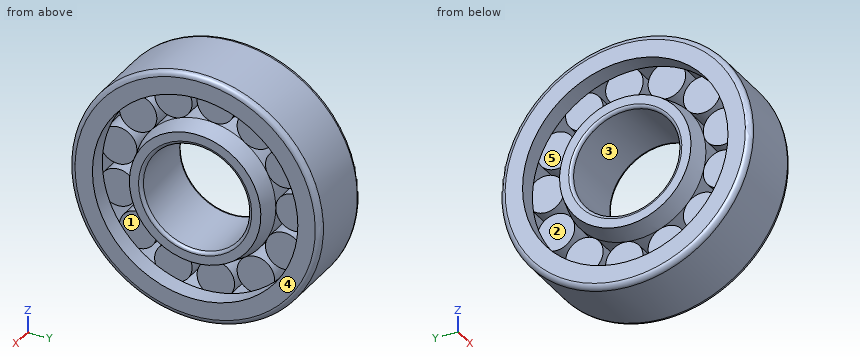
from build123d import *

# Parameters (mm, degrees)
SKETCH2_W               = 7
SKETCH2_H               = 3.51
CIRCULAR_PATTERN1_COUNT = 13
FILLET1_R               = 1
FILLET2_R               = 0.6


with BuildPart() as part:
    # Sketch1 → Revolve1 (revolve)
    with BuildSketch(Plane.XY, mode=Mode.PRIVATE) as revolve1_sk:
        Polygon((-7, 10), (7, 10), (7, 12.312177826), (3.5, 13.25), (-3.5, 13.25), (-7, 12.312177826), align=None)
    revolve(revolve1_sk.sketch.rotate(Axis((-10.137871204, 0, 0), (1, 0, 0)), 90), axis=Axis((-10.137871204, 0, 0), (1, 0, 0)))

    # Sketch2 → Revolve2 (revolve)
    with BuildSketch(Plane.XY):
        with Locations((0, 14.995)):
            Rectangle(SKETCH2_W, SKETCH2_H)
    revolve2 = revolve(axis=Axis((-7.422783257, 16.75, 0), (1, 0, 0)))

    # Sketch3 → Revolve3 (revolve)
    with BuildSketch(Plane.XY, mode=Mode.PRIVATE) as revolve3_sk:
        Polygon((-7, 23.5), (7, 23.5), (7, 19.2375), (3.49, 19.2375), (3.49, 20.25), (-3.49, 20.25), (-3.49, 19.2375), (-7, 19.2375), align=None)
    revolve(revolve3_sk.sketch.rotate(Axis((-9.082213196, 0, 0), (1, 0, 0)), 90), axis=Axis((-9.082213196, 0, 0), (1, 0, 0)))

    # Circular-Pattern1: Revolve2 ×13 about axis
    circular_pattern1_axis = Axis((0, 0, 0), (1, 0, 0))
    for i in range(1, CIRCULAR_PATTERN1_COUNT):
        add(revolve2.rotate(circular_pattern1_axis, i * 360 / CIRCULAR_PATTERN1_COUNT))

    # Fillet1
    fillet1_edges = [part.edges().sort_by_distance(p)[0] for p in [
        (-7, 0, -23.5),
        (7, 0, -23.5),
    ]]
    fillet(fillet1_edges, radius=FILLET1_R)

    # Fillet2
    fillet2_edges = [part.edges().sort_by_distance(p)[0] for p in [
        (7, 0, -10),
        (-7, 0, -10),
    ]]
    fillet(fillet2_edges, radius=FILLET2_R)


solid = part.part
Could you check a few things on this model? Use its own coordinates, in mm. Face numbers are marked on the shaded views. A direction names the side the tool comes from. Give positions to 0.01 mm unless a question says otherwise; leave off trailing zeros. One line per question, with ' | ' between items.
1. I'm going to push flat-ended pins straight in: pin 1 (5.5 mm diameter, centred on y = -12.5, z = -10.5, fed in from -X); pin 2 (3.5 mm diameter, centred on y = 10, z = 12.5, fed in from +X); pin 3 (1 mm diameter, centred on x = 2.5, z = 9, fed in from -Y). Where does each tip first touch, or does it pass through?
Results:
pin 1: x = -3.5 | pin 2: x = 3.5 | pin 3: y = -21.91
2. For the marked faces 1, 2 and 3, which set-ups out of +Z, -Z, +X, -X, +Y, -Y let a thin tool reach every point of the face, with its end or its side?
Results:
face 1: +X | face 2: -X | face 3: +X, -X
3. If I drill on line 1 (Z direction, x = 4.75, y = -5); line 2 (Y direction, x = 4.9, z = 0); line 3 (Z direction, x = 3.75, y = 5), over which ranges is the centre line in solid material (lowest first)?
Results:
line 1: -22.96 to -18.58, -11.91 to -8.66, 8.66 to 11.91, 18.58 to 22.96 | line 2: -23.5 to -19.24, -12.87 to -10, 10 to 12.87, 19.24 to 23.5 | line 3: -22.96 to -18.58, -12.2 to -8.66, 8.66 to 12.2, 18.58 to 22.96
4. I want a section at A-A (y = 14.5). Give the number of separate pieces and of enclosed holes in the cut face, and give its area (3 significant figures).
Results:
separate pieces: 5 | enclosed holes: 0 | area: 277 mm²
5. We'd pull the mould along Y, two halves only. Please class the marked faces 4 and 5: +Y half, -Y half, draft (parallel to the pull), parting line (faces both ways), or undercut.
Results:
face 4: draft | face 5: undercut
